Part print with two shaded views. Sizes in mm from the minimum x, y, z corner. A direction names the side the tool comes from. Coordinates: 2 decimals unless noted, no trailing zeros. Loops run counter-clockwise (first coordinate to the right, second up) from the corner with the lowest first, then second, coordinate; pieces in that order, holes last. Notation, with made-up numbers: M -12.5,59 L 40.5,59 A15 cw 40.5,83 Z; hole C -3.5,42 d1. An arc over 180 degrees is marked long. Use CSV: the item, a comma, the result in double quotes. Start each with the question number.
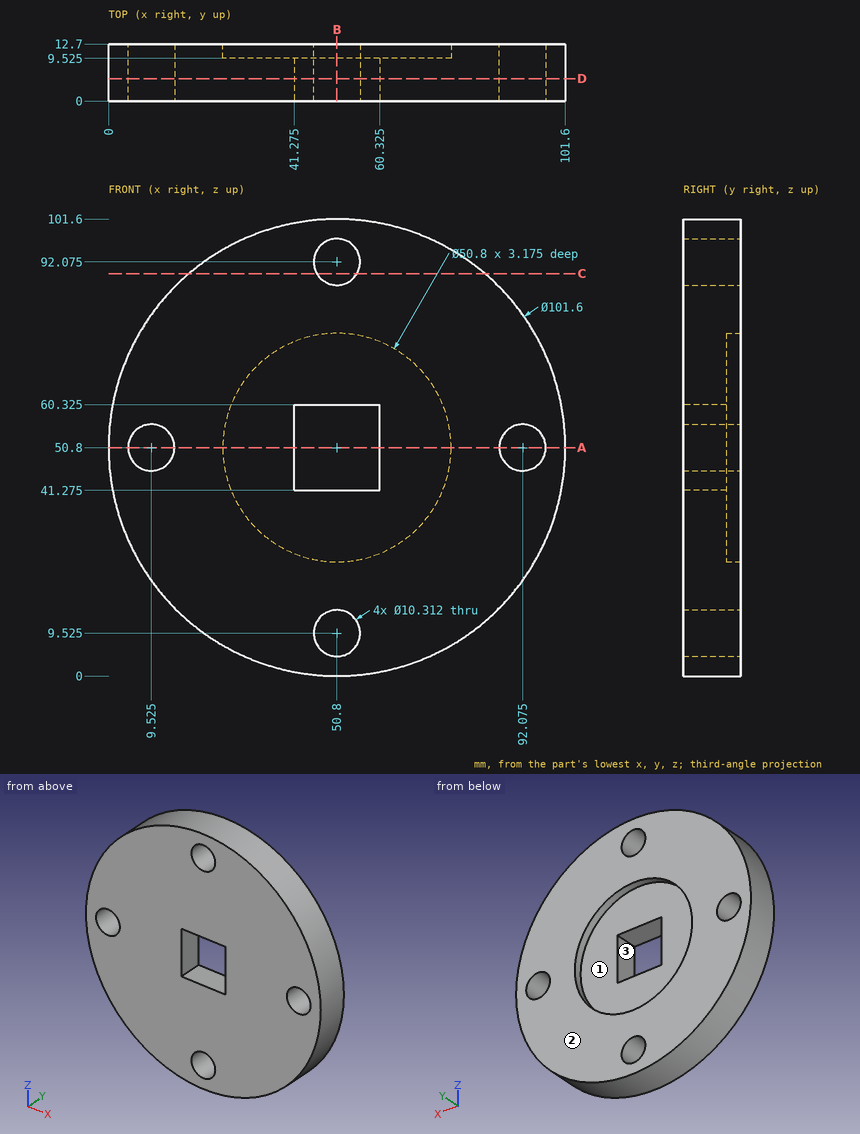
1. Pin check, flat tips, straight feed: pin 1 (1 mm diameter, centred on x = 44, y = 7, fed in from +Z); pin 2 (9.5 mm diameter, centred on x = 9.525, z = 50.8, fed in from +Y); pin 3 (1.5 mm diameter, centred on y = 9, z = 55.5, fed in from -X); pin 4 (3 mm diameter, centred on x = 12.5, y = 4.5, fed in from +Z). Stop position of each tip, or through.
2. Slice it at D-D, the plane y = 5. List the corners of the cut face in (x, z) (1 decimal), and give its area (3 significant figures).
3. Slice it at B-B, the plane x = 50.8. List the corners of the cut face in (y, z) (1 decimal).
4. Wall check: probe 1 along Z at (x, y) = (50.8, 4.5) (1 decimal); probe 2 along Z at (x, y) = (50.8, 11.3); probe 3 along Z at (x, y) = (27.5, 10.75) (1 decimal). Give the ranges that are in metal, low to high.
5. Tool access for the marked faces 1, 2 and 3: list every direction of +Z, -Z, +X, -X, +Y, -Y with a clear straight run to the whole face (end or side of a thin tool).
6. Slice it at A-A, the plane z = 50.8. List the corners of the cut face in (x, y) (1 decimal).
7. Slice it at C-C, the plane z = 89.5. List the corners of the cut face in (x, y).
Found:
1,pin 1,"z = 101.21"
1,pin 2,"through"
1,pin 3,"x = 0.15"
1,pin 4,"z = 85.82"
2,outline,"C 50.8,50.8 d101.6; hole C 9.5,50.8 d10.3; hole M 41.3,41.3 L 60.3,41.3 L 60.3,60.3 L 41.3,60.3 Z; hole C 50.8,9.5 d10.3; hole C 50.8,92.1 d10.3; hole C 92.1,50.8 d10.3"
2,area,"7,410 mm^2"
3,outline,"M 0,0 L 12.7,0 L 12.7,4.4 L 0,4.4 Z; M 0,14.7 L 12.7,14.7 L 12.7,25.4 L 9.5,25.4 L 9.5,41.3 L 0,41.3 Z; M 0,60.3 L 9.5,60.3 L 9.5,76.2 L 12.7,76.2 L 12.7,86.9 L 0,86.9 Z; M 0,97.2 L 12.7,97.2 L 12.7,101.6 L 0,101.6 Z"
4,probe 1,"0 to 4.4, 14.7 to 41.3, 60.3 to 86.9, 97.2 to 101.6"
4,probe 2,"0 to 4.37, 14.68 to 25.4, 76.2 to 86.92, 97.23 to 101.6"
4,probe 3,"5.7 to 40.7, 60.9 to 95.9"
5,face 1,"+Y"
5,face 2,"+Z, -Z, +X, -X, +Y"
5,face 3,"+Y, -Y"
6,outline,"M 0,0 L 4.4,0 L 4.4,12.7 L 0,12.7 Z; M 14.7,0 L 41.3,0 L 41.3,9.5 L 25.4,9.5 L 25.4,12.7 L 14.7,12.7 Z; M 60.3,0 L 86.9,0 L 86.9,12.7 L 76.2,12.7 L 76.2,9.5 L 60.3,9.5 Z; M 97.2,0 L 101.6,0 L 101.6,12.7 L 97.2,12.7 Z"
7,outline,"M 17.89,0 L 46.33,0 L 46.33,12.7 L 17.89,12.7 Z; M 55.27,0 L 83.71,0 L 83.71,12.7 L 55.27,12.7 Z"
